from build123d import *

# Parameters (mm, degrees)
SKETCH_1_W          = 10
SKETCH_1_H          = 10
EXTRUDE_1_DEPTH     = 10
CUT_EXTRUDE_1_DEPTH = 2.1


with BuildPart() as part:
    # Sketch 1 → Extrude 1 (new body)
    with BuildSketch(Plane.XY):
        with Locations((5, 5)):
            Rectangle(SKETCH_1_W, SKETCH_1_H)
    extrude(amount=EXTRUDE_1_DEPTH)

    # Sketch 2 → Cut-Extrude 1 (cut)
    with BuildSketch(Plane(origin=(0, 50, 0), x_dir=(1, 0, 0), z_dir=(0, 0, 1))):
        Polygon((5, -41.824573519), (2.25, -43.41228676), (2.25, -46.58771324), (5, -48.175426481), (7.75, -46.58771324), (7.75, -43.41228676), align=None)
    extrude(amount=CUT_EXTRUDE_1_DEPTH, mode=Mode.SUBTRACT)


solid = part.part
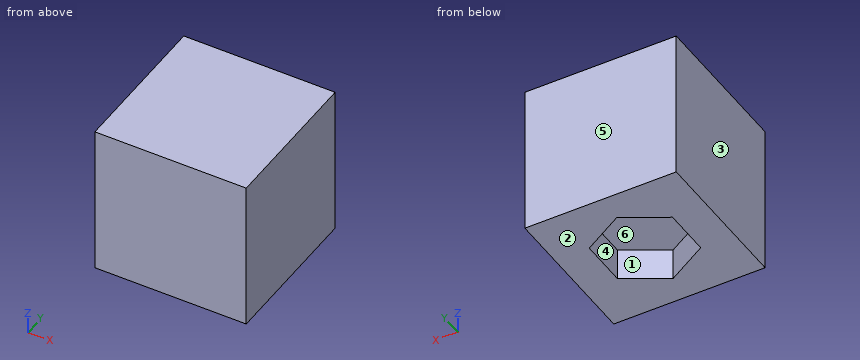
Here's how the part is built. I have some questions about the finished solid (model axes, mm). Face numbers are marked on the shaded views. A direction names the side the tool comes from. Round coordinates to 2 decimals unless told otherwise and drop trailing zeros. Write each loop counter-clockwise with the first axis right and the second up, starting at its lowest first coordinate (ties: lowest second). Pieces come first, ordered by that corner, then holes.
1. If we mould it in two halves opening along X, with no side actions, what happens to the marked faces 1, 2, 3 and 4? For each: released by +X, released by -X, zero draft, split by the parting line, or undercut.
2. I need wall thicknesses on L1, parallel to Z at x = 4, y = 4.75; L2, parallel to X at y = 4.75, z = 2; L3, parallel to X at y = 7.75, z = 1. Which ranges of each line are inside material? Lowest first, please.
3. Suppose I cut it at C-C (x = 4.25). List the corners of the cut face in (y, z) for me.
4. Suppose I cut it at B-B (y = 6). List the corners of the cut face in (x, z) for me.
5. Suppose I cut it at A-A (z = 1). List the corners of the cut face in (x, y) for me, and give its area (3 significant figures).
6. For the marked faces 5 and 6, which set-ups out of +Z, -Z, +X, -X, +Y, -Y let a thin tool reach every point of the face, with its end or its side?
7. Will this pin go through, and if not, where does the flat tip stop? pin 1 Ø3 at (x, y) = (5, 3.5) entering from -Z.
Answer sheet:
1. face 1: undercut
1. face 2: zero draft
1. face 3: released by -X
1. face 4: undercut
2. L1: z = 2.1 to 10
2. L2: x = 0 to 2.25, 7.75 to 10
2. L3: x = 0 to 4.26, 5.74 to 10
3. outline: (0, 0) - (2.26, 0) - (2.26, 2.1) - (7.74, 2.1) - (7.74, 0) - (10, 0) - (10, 10) - (0, 10) - close
4. outline: (0, 0) - (2.25, 0) - (2.25, 2.1) - (7.75, 2.1) - (7.75, 0) - (10, 0) - (10, 10) - (0, 10) - close
5. outline: (0, 0) - (10, 0) - (10, 10) - (0, 10) - close; hole (2.25, 3.41) - (5, 1.82) - (7.75, 3.41) - (7.75, 6.59) - (5, 8.18) - (2.25, 6.59) - close
5. area: 73.8 mm2
6. face 5: +Z, -Z, +X, -X, +Y
6. face 6: -Z
7. pin 1: stops at z = 0
